Check sheet for the modelled part. Datum: model origin and axes. Units: mm. A direction names the side the tool comes from. Coordinates: 2 decimals unless noted, no trailing zeros. Order: outer loops, then holes, each group sorted by start corner. A loop starts at its lowest first (then second) coordinate and runs counter-clockwise, first axis right, second up.
from build123d import *

# Parameters (mm, degrees)
SKETCH2_W          = 16
SKETCH2_H          = 14
CUT_EXTRUDE1_DEPTH = 110.5


with BuildPart() as part:
    # Sketch1 → Revolve1 (revolve)
    with BuildSketch(Plane.XY):
        with BuildLine():
            Line((-28, 0), (-28, 46))
            Line((-28, 46), (-32, 50))
            Line((-32, 50), (-47, 50))
            Line((-47, 50), (-47, 47))
            Line((-47, 47), (-53.5, 47))
            ThreePointArc((-53.5, 47), (-55.621320344, 47.878679656), (-56.5, 50))
            Line((-56.5, 50), (-56.5, 75))
            Line((-56.5, 75), (-62.5, 75))
            Line((-62.5, 75), (-62.5, 47))
            ThreePointArc((-62.5, 47), (-61.035533906, 43.464466094), (-57.5, 42))
            Line((-57.5, 42), (-43.94, 42))
            Line((-43.94, 42), (-43.94, 2))
            Line((-43.94, 2), (-41.94, 0))
            Line((-41.94, 0), (-28, 0))
        make_face()
    revolve(axis=Axis((0, 0, 0), (0, 1, 0)))

    # Sketch2 → Cut-Extrude1 (cut, symmetric)
    with BuildSketch(Plane.XY):
        with Locations((0, 68)):
            Rectangle(SKETCH2_W, SKETCH2_H)
    extrude(amount=CUT_EXTRUDE1_DEPTH, both=True, mode=Mode.SUBTRACT)


solid = part.part
(1) Thickness scan on probe 1 along X at (y, z) = (58, 0); probe 2 along Z at (x, y) = (0, 25.5); probe 3 along Y at (x, z) = (-38, 9.5). Record the ranges inside material, lowest first.
Filled in:
probe 1: x = -62.5 to -56.5, 56.5 to 62.5
probe 2: z = -43.94 to -28, 28 to 43.94
probe 3: y = 0 to 50
(2) Cross-section at C-C (y = 58.5). Enter the section's corners in (x, z), and give its area (3 significant figures).
Filled in:
outline: circle Ø125 at (0, 0); hole circle Ø113 at (0, 0)
area: 2,240 mm2
(3) Tool access check on faces 4 (the flat face through (13, 42, -42.3)), 5 (the flat face through (-8, 68, 59)), 6 (the flat face through (10, 50, -31)). Record the directions out of +Z, -Z, +X, -X, +Y, -Y that give a thin tool (end or side, any length) a straight path to the whole face; none if there is none.
Filled in:
face 4: -Y
face 5: +Z, -Z, +Y
face 6: +Y
(4) Cross-section at B-B (z = 0). Enter the section's corners in (x, y), and give its area (3 significant figures).
Filled in:
outline: (-62.5, 47) arc R5 ccw to (-57.5, 42) - (-43.94, 42) - (-43.94, 2) - (-41.94, 0) - (-28, 0) - (-28, 46) - (-32, 50) - (-47, 50) - (-47, 47) - (-53.5, 47) arc R3 cw to (-56.5, 50) - (-56.5, 75) - (-62.5, 75) - close; (28, 0) - (41.94, 0) - (43.94, 2) - (43.94, 42) - (57.5, 42) arc R5 ccw to (62.5, 47) - (62.5, 75) - (56.5, 75) - (56.5, 50) arc R3 cw to (53.5, 47) - (47, 47) - (47, 50) - (32, 50) - (28, 46) - close
area: 2,110 mm2
(5) Cross-section at A-A (x = 0). Enter the section's corners in (y, z), and give its area (3 significant figures).
Filled in:
outline: (0, -41.94) - (2, -43.94) - (42, -43.94) - (42, -57.5) arc R5 ccw to (47, -62.5) - (61, -62.5) - (61, -56.5) - (50, -56.5) arc R3 cw to (47, -53.5) - (47, -47) - (50, -47) - (50, -32) - (46, -28) - (0, -28) - close; (0, 28) - (46, 28) - (50, 32) - (50, 47) - (47, 47) - (47, 53.5) arc R3 cw to (50, 56.5) - (61, 56.5) - (61, 62.5) - (47, 62.5) arc R5 ccw to (42, 57.5) - (42, 43.94) - (2, 43.94) - (0, 41.94) - close
area: 1,940 mm2
(6) Release check for a two-part mould opening along Z. For faces 1 (the flat face through (-27, 0, -9)), 2 (the cylindrical face through (9.5, 21.7, -42.9)), 3 (the cylindrical face through (-26.071, 62.675, -50.125)) record: +Z half, -Z half, draft (parallel to the pull), parting line (faces both ways), or undercut.
Filled in:
face 1: draft
face 2: parting line
face 3: undercut
(7) Cross-section at D-D (y = 26). Enter the section's corners in (x, z), and give its area (3 significant figures).
Filled in:
outline: circle Ø87.88 at (0, 0); hole circle Ø56 at (0, 0)
area: 3,600 mm2
(8) Go/stop test with flat-tipped pins: P1, Ø3, axis at y = 70, z = -59, coming from the -X side; P2, Ø1.5, axis at x = -15, y = 22.5, coming from the +Z side; P3, Ø2, axis at x = -3, z = -58, coming from the +Y side; P4, Ø8, axis at x = 10.5, z = -29, coming from the -Y side. Record where each tip stops, or that it passes through.
Filled in:
P1: stops at x = -24.49
P2: stops at z = 41.57
P3: stops at y = 61
P4: stops at y = 0
